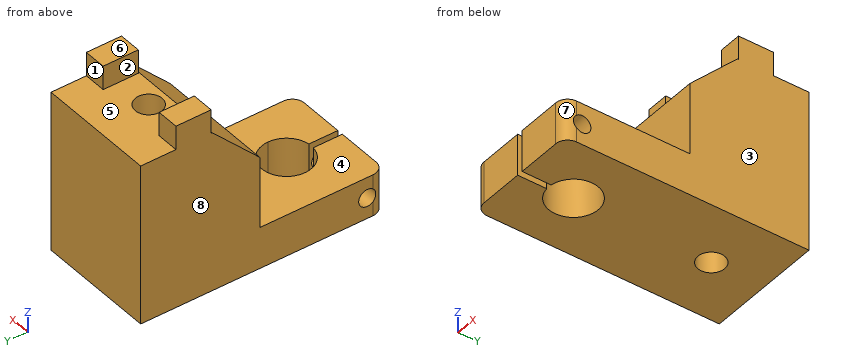
```python
from build123d import *

# Parameters (mm, degrees)
F1_DEPTH    = 7
F2_R        = 1.45
F3_DEPTH    = 25
F4_T1_DEPTH = 17
F5_DEPTH    = 27
F0_W        = 3.75
F0_H        = 5.9
F6_DEPTH    = 31
F7_SIZE     = 8


# Not quite as in the source:
# - a fillet or chamfer that OpenCascade refuses, or shapes differently, is made with other operations: its cross-section is extruded or revolved along the edge and cut away or added


with BuildPart() as f1:
    # F0 (on Top) → F1 (new body)
    with BuildSketch(Plane.XY):
        with BuildLine():
            Line((-6.5963959517, 29.175), (-6.5963959517, 21))
            Line((-6.5963959517, 21), (3.4036040483, 21))
            Line((3.4036040483, 21), (3.4036040483, 29.875))
            ThreePointArc((3.4036040483, 29.875), (1.8126137907, 30.5340097423), (1.1536040483, 32.125))
            ThreePointArc((1.1536040483, 32.125), (1.8126137907, 33.7159902577), (3.4036040483, 34.375))
            Line((3.4036040483, 34.375), (3.4036040483, 41))
            Line((3.4036040483, 41), (-6.5963959517, 41))
            Line((-6.5963959517, 41), (-6.5963959517, 35.075))
            Line((-6.5963959517, 35.075), (-2.8463959517, 35.075))
            Line((-2.8463959517, 35.075), (-2.8463959517, 29.175))
            Line((-2.8463959517, 29.175), (-6.5963959517, 29.175))
        make_face()
        with BuildLine():
            Line((3.4036040483, 29.875), (3.4036040483, 21))
            Line((3.4036040483, 21), (13.4036040483, 21))
            Line((13.4036040483, 21), (13.4036040483, 29.175))
            Line((13.4036040483, 29.175), (9.6536040483, 29.175))
            Line((9.6536040483, 29.175), (9.6536040483, 35.075))
            Line((9.6536040483, 35.075), (13.4036040483, 35.075))
            Line((13.4036040483, 35.075), (13.4036040483, 41))
            Line((13.4036040483, 41), (3.4036040483, 41))
            Line((3.4036040483, 41), (3.4036040483, 34.375))
            ThreePointArc((3.4036040483, 34.375), (4.994594306, 33.7159902577), (5.6536040483, 32.125))
            ThreePointArc((5.6536040483, 32.125), (4.994594306, 30.5340097423), (3.4036040483, 29.875))
        make_face()
        with BuildLine():
            Line((-6.5963959517, 21), (-6.5963959517, 0))
            Line((-6.5963959517, 0), (2.9036040483, 0))
            Line((2.9036040483, 0), (2.9036040483, 1.2661458509))
            ThreePointArc((2.9036040483, 1.2661458509), (-1.8967497135, 14.6540914389), (11.1536040483, 9))
            ThreePointArc((11.1536040483, 9), (9.0576954873, 3.6996462382), (3.9036040483, 1.2661458509))
            Line((3.9036040483, 1.2661458509), (3.9036040483, 0))
            Line((3.9036040483, 0), (13.4036040483, 0))
            Line((13.4036040483, 0), (13.4036040483, 21))
            Line((13.4036040483, 21), (3.4036040483, 21))
            Line((3.4036040483, 21), (-6.5963959517, 21))
        make_face()
        with BuildLine():
            ThreePointArc((11.1536040483, 9), (-1.8967497135, 14.6540914389), (2.9036040483, 1.2661458509))
            Line((2.9036040483, 1.2661458509), (2.9036040483, 4.880230589))
            ThreePointArc((2.9036040483, 4.880230589), (0.6515593539, 12.1062437123), (7.5536040483, 9))
            ThreePointArc((7.5536040483, 9), (6.5098477606, 6.2479553056), (3.9036040483, 4.880230589))
            Line((3.9036040483, 4.880230589), (3.9036040483, 1.2661458509))
            ThreePointArc((3.9036040483, 1.2661458509), (9.0576954873, 3.6996462382), (11.1536040483, 9))
        make_face()
    extrude(amount=F1_DEPTH)

    # F2 (on face) → F3 (cut)
    with BuildSketch(Plane.YZ.offset(13.4036040483)):
        with Locations((2.95, 3.5)):
            Circle(F2_R)
    extrude(amount=-F3_DEPTH, mode=Mode.SUBTRACT)

    # F4: fillet of radius 2 on 2 edges, made by hand

    # F4_s2 → F4_t1 (cut)
    with BuildSketch(Plane.XY.offset(-5)):
        with BuildLine():
            ThreePointArc((11.4036040483, 0), (12.8178176107, 0.5857864376), (13.4036040483, 2))
            Line((13.4036040483, 2), (13.4036040483, 0))
            Line((13.4036040483, 0), (11.4036040483, 0))
        make_face()
        with BuildLine():
            ThreePointArc((-6.5963959517, 2), (-6.010609514, 0.5857864376), (-4.5963959517, 0))
            Line((-4.5963959517, 0), (-6.5963959517, 0))
            Line((-6.5963959517, 0), (-6.5963959517, 2))
        make_face()
    extrude(amount=F4_T1_DEPTH, mode=Mode.SUBTRACT)

    # F0 (on Top) → F5 (join)
    with BuildSketch(Plane.XY):
        with BuildLine():
            Line((3.4036040483, 29.875), (3.4036040483, 21))
            Line((3.4036040483, 21), (13.4036040483, 21))
            Line((13.4036040483, 21), (13.4036040483, 29.175))
            Line((13.4036040483, 29.175), (9.6536040483, 29.175))
            Line((9.6536040483, 29.175), (9.6536040483, 35.075))
            Line((9.6536040483, 35.075), (13.4036040483, 35.075))
            Line((13.4036040483, 35.075), (13.4036040483, 41))
            Line((13.4036040483, 41), (3.4036040483, 41))
            Line((3.4036040483, 41), (3.4036040483, 34.375))
            ThreePointArc((3.4036040483, 34.375), (4.994594306, 33.7159902577), (5.6536040483, 32.125))
            ThreePointArc((5.6536040483, 32.125), (4.994594306, 30.5340097423), (3.4036040483, 29.875))
        make_face()
        with BuildLine():
            Line((-6.5963959517, 29.175), (-6.5963959517, 21))
            Line((-6.5963959517, 21), (3.4036040483, 21))
            Line((3.4036040483, 21), (3.4036040483, 29.875))
            ThreePointArc((3.4036040483, 29.875), (1.8126137907, 30.5340097423), (1.1536040483, 32.125))
            ThreePointArc((1.1536040483, 32.125), (1.8126137907, 33.7159902577), (3.4036040483, 34.375))
            Line((3.4036040483, 34.375), (3.4036040483, 41))
            Line((3.4036040483, 41), (-6.5963959517, 41))
            Line((-6.5963959517, 41), (-6.5963959517, 35.075))
            Line((-6.5963959517, 35.075), (-2.8463959517, 35.075))
            Line((-2.8463959517, 35.075), (-2.8463959517, 29.175))
            Line((-2.8463959517, 29.175), (-6.5963959517, 29.175))
        make_face()
    extrude(amount=F5_DEPTH)

    # F0 (on Top) → F6 (join)
    with BuildSketch(Plane.XY):
        with Locations((-4.7213959517, 32.125)):
            Rectangle(F0_W, F0_H)
        with Locations((11.5286040483, 32.125)):
            Rectangle(F0_W, F0_H)
    extrude(amount=F6_DEPTH)

    # F7
    f7_edges = [f1.edges().sort_by_distance(p)[0] for p in [
        (3.403604, 21, 27),
    ]]
    chamfer(f7_edges, length=F7_SIZE)


solid = f1.part
```
Geometry check sheet. Reference: the model listing, model coordinates, mm. Face numbers are marked on the shaded views. A direction names the side the tool comes from. Coordinates: 2 decimals unless noted, no trailing zeros. Write each loop counter-clockwise with the first axis right and the second up, starting at its lowest first coordinate (ties: lowest second). Pieces come first, ordered by that corner, then holes. Notation, with made-up numbers: M 10.25,-39 L 31.25,-39 A26 ccw 31.25,-22 Z; hole C 8.25,9.25 d2. An arc over 180 degrees is marked long. Use one line per item in the form item = value. Start each with the question number.
1) Section check D-D on y = 23.5. Enter the section's corners in (x, z), and give its area (3 significant figures).
2) Release check for a two-part mould opening along X. For the marked faces 5, 6, 7 and 8 record: pulls with the +X half, pulls with the -X half, needs draft (parallel to the pull), parting line crosses it, or undercut.
3) Set-up check for the marked faces 1, 2, 3 and 4: record each of +Z, -Z, +X, -X, +Y, -Y from which the full face is reachable in a straight line by a thin tool's end or side.
4) Section check B-B on y = 2.95. Enter the section's corners in (x, z), and give its area (3 significant figures).
5) Section check C-C on x = 9. Enter the section's corners in (y, z), and give its area (3 significant figures).
6) Section check A-A on z = 3.5. Enter the section's corners in (x, y) (3 decimals).
7) Thickness scan on probe 1 along X at (y, z) = (9, 4.5); probe 2 along Y at (x, z) = (12.25, 16.5); probe 3 along Z at (x, y) = (-4.25, 13). Record the ranges inside material, lowest first. Write a range as from..to.
8) Go/stop test with flat-tipped pins: pin 1 Ø1.9 at (x, z) = (10.5, 29) entering from -Y (3 decimals); pin 2 Ø2 at (x, y) = (0.5, 14.5) entering from +Z; pin 3 Ø3.5 at (x, z) = (7.5, 11.5) entering from -Y. Record where each tip stops, or that it passes through.
Responses:
q1.outline = M -6.6,0 L 13.4,0 L 13.4,21.5 L -6.6,21.5 Z
q1.area = 430 mm2
q2.face_5 = undercut
q2.face_6 = needs draft
q2.face_7 = pulls with the +X half
q2.face_8 = pulls with the -X half
q3.face_1 = +Z, +X, -X, +Y
q3.face_2 = +Z, +Y, -Y
q3.face_3 = +Z, -Z, +X, +Y, -Y
q3.face_4 = +Z, +X, -X, -Y
q4.outline = M -6.6,0 L 2.9,0 L 2.9,2.05 L -6.6,2.05 Z; M -6.6,4.95 L 2.9,4.95 L 2.9,7 L -6.6,7 Z; M 3.9,0 L 13.4,0 L 13.4,2.05 L 3.9,2.05 Z; M 3.9,4.95 L 13.4,4.95 L 13.4,7 L 3.9,7 Z
q4.area = 77.9 mm2
q5.outline = M 0,0 L 41,0 L 41,27 L 29,27 L 21,19 L 21,7 L 0,7 Z; hole C 2.95,3.5 d2.9
q5.area = 648 mm2
q6.outline = M -6.596,4.4 L 2.904,4.4 L 2.904,4.88 A4.15 cw long 3.904,4.88 L 3.904,4.4 L 13.404,4.4 L 13.404,41 L -6.596,41 Z; M -6.533,1.5 A2 ccw -4.596,0 L 2.904,0 L 2.904,1.5 Z; M 3.904,0 L 11.404,0 A2 ccw 13.34,1.5 L 3.904,1.5 Z; hole C 3.404,32.125 d4.5
q7.probe_1 = -6.6..-0.75, 7.55..13.4
q7.probe_2 = 21..41
q7.probe_3 = 0..7
q8.pin_1 = 29.175
q8.pin_2 = 7
q8.pin_3 = 21
